Verification items for the finished model (mm, model axes). A direction names the side the tool comes from. Give positions to 0.01 mm unless a question says otherwise; leave off trailing zeros. Loops run counter-clockwise (first coordinate to the right, second up) from the corner with the lowest first, then second, coordinate; pieces in that order, holes last. Notation, with made-up numbers: (49, 25) -> (75, 25) arc R14 cw to (75, 43) -> close; hole circle Ø4 at (2.5, 65). An arc over 180 degrees is marked (long way). Answer in a Markdown table with one row per item. Add a question column.
Q1. Set-up check for faces 1 (the face through (0, 2, 39.688)), 2 (the face through (-2, 10, -1)): record each of +Z, -Z, +X, -X, +Y, -Y from which the full face is reachable in a straight line by a thin tool's end or side.
Q2. Material ranges on probe 1 along Y at (x, z) = (-16.5, -31); probe 2 along X at (y, z) = (18.5, 7), recorded low to high.
Q3. Section check C-C on z = -33. Enter the section's corners in (x, y), and give its area (3 significant figures).
Q4. Section check A-A on x = 5. Enter the section's corners in (y, z), and give its area (3 significant figures).
Q5. Section check B-B on y = 11.25. Enter the section's corners in (x, z), and give its area (3 significant figures).
Q6. Gauge pin test, flat ends, axial feed: P1, Ø4, axis at x = 9, z = -30, coming from the +Y side; P2, Ø10, axis at x = 6.5, y = 14.5, coming from the -Z side. Record the tip position at first contact, or that the pin passes through.
```python
from build123d import *

# Parameters (mm, degrees)
BOSS_EXTRUDE1_DEPTH      = 39.6875
BOSS_EXTRUDE1_DEPTH_BACK = 39.6875


with BuildPart() as part:
    # Sketch1 → Boss-Extrude1 (new, two sides: drawn at the far end of the back side and taken through both)
    with BuildSketch(Plane.XY.offset(-BOSS_EXTRUDE1_DEPTH_BACK)):
        Polygon((-20, 10), (17, 10), (17, 20), (20, 20), (20, 10), (20, -10), (-20, -10), align=None)
    extrude(amount=BOSS_EXTRUDE1_DEPTH + BOSS_EXTRUDE1_DEPTH_BACK)


solid = part.part
```
Taken from the geometry:
| question | item | result |
|---|---|---|
| 1 | face 1 | +Z, +X, -X, +Y, -Y |
| 1 | face 2 | +Z, -Z, -X, +Y |
| 2 | probe 1 | y = -10 to 10 |
| 2 | probe 2 | x = 17 to 20 |
| 3 | outline | (-20, -10) -> (20, -10) -> (20, 20) -> (17, 20) -> (17, 10) -> (-20, 10) -> close |
| 3 | area | 830 mm² |
| 4 | outline | (-10, -39.69) -> (10, -39.69) -> (10, 39.69) -> (-10, 39.69) -> close |
| 4 | area | 1,590 mm² |
| 5 | outline | (17, -39.69) -> (20, -39.69) -> (20, 39.69) -> (17, 39.69) -> close |
| 5 | area | 238 mm² |
| 6 | P1 | stops at y = 10 |
| 6 | P2 | stops at z = -39.69 |
